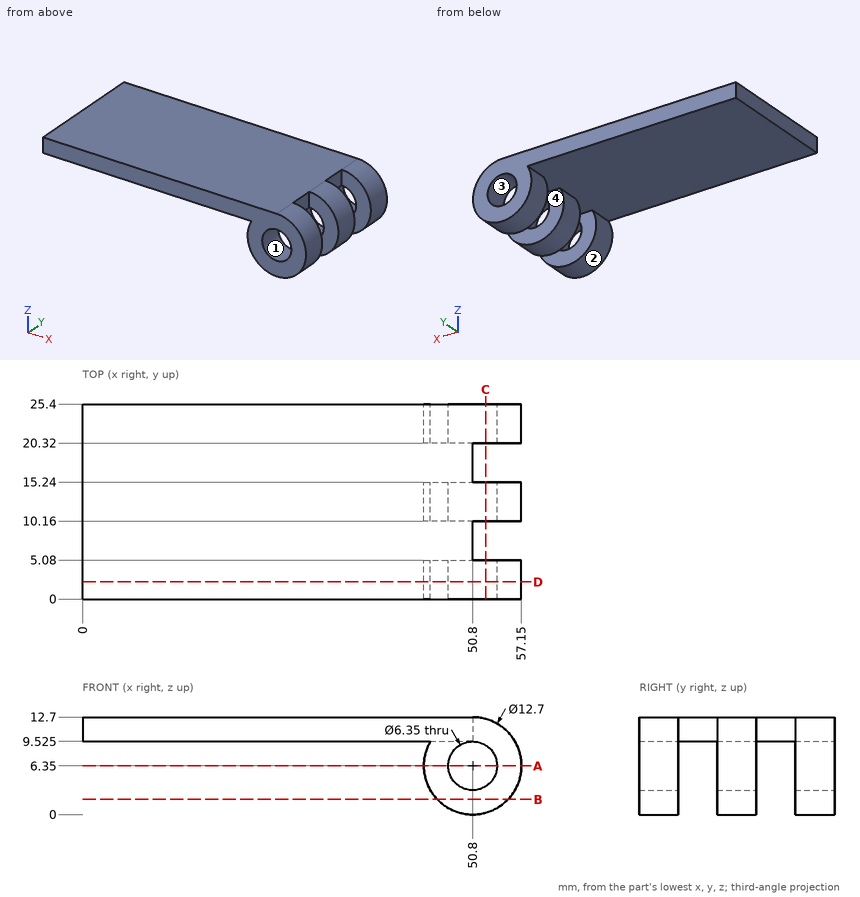
Part print with two shaded views. Sizes in mm from the minimum x, y, z corner. Round coordinates to 2 decimals unless told otherwise and drop trailing zeros. Loops run counter-clockwise (first coordinate to the right, second up) from the corner with the lowest first, then second, coordinate; pieces in that order, holes last.
Item 1: Saw through at D-D (y = 2.25). List the corners of the cut face in (x, z) (3 decimals), then the cut area to 3 significant figures.
Item 2: Saw through at C-C (x = 52.5). List the corners of the cut face in (y, z), then the cut area to 3 significant figures.
Item 3: Drill centre lines: line 1 along X through (y, z) = (3.5, 6.35) (3 decimals); line 2 along Z through (x, y) = (9, 6) (3 decimals); line 3 along X through (y, z) = (24, 9). Where is each one in solid material? Low to high.
Item 4: Saw through at A-A (z = 6.35). List the corners of the cut face in (x, y) (3 decimals).
Item 5: Pin check, flat tips, straight feed: P1, Ø4, axis at x = 45, z = 4.5, coming from the -Y side; P2, Ø1, axis at y = 6.5, z = 11.5, coming from the +X side; P3, Ø4, axis at y = 12, z = 6.5, coming from the -X side; P4, Ø4, axis at y = 15.5, z = 3, coming from the -X side. Stop position of each tip, or through.
Item 6: Two-plate mould, pull along X, no slides. Class the marked faces 1, 2, 3 and 4: released by +X, released by -X, zero draft, split by the parting line, or undercut.
Item 7: Saw through at B-B (z = 2). List the corners of the cut face in (x, y).
Worked answers:
1. outline: (0, 9.525) - (45.301, 9.525) arc R6.35 ccw (long way) to (50.8, 12.7) - (0, 12.7) - close; hole circle Ø6.35 at (50.8, 6.35)
1. area: 244 mm2
2. outline: (0, 0.23) - (5.08, 0.23) - (5.08, 3.67) - (0, 3.67) - close; (0, 9.03) - (5.08, 9.03) - (5.08, 12.47) - (0, 12.47) - close; (10.16, 0.23) - (15.24, 0.23) - (15.24, 3.67) - (10.16, 3.67) - close; (10.16, 9.03) - (15.24, 9.03) - (15.24, 12.47) - (10.16, 12.47) - close; (20.32, 0.23) - (25.4, 0.23) - (25.4, 3.67) - (20.32, 3.67) - close; (20.32, 9.03) - (25.4, 9.03) - (25.4, 12.47) - (20.32, 12.47) - close
2. area: 105 mm2
3. line 1: x = 44.45 to 47.625, 53.975 to 57.15
3. line 2: z = 9.525 to 12.7
3. line 3: x = 45.03 to 49.05, 52.55 to 56.57
4. outline: (44.45, 0) - (47.625, 0) - (47.625, 5.08) - (44.45, 5.08) - close; (44.45, 10.16) - (47.625, 10.16) - (47.625, 15.24) - (44.45, 15.24) - close; (44.45, 20.32) - (47.625, 20.32) - (47.625, 25.4) - (44.45, 25.4) - close; (53.975, 0) - (57.15, 0) - (57.15, 5.08) - (53.975, 5.08) - close; (53.975, 10.16) - (57.15, 10.16) - (57.15, 15.24) - (53.975, 15.24) - close; (53.975, 20.32) - (57.15, 20.32) - (57.15, 25.4) - (53.975, 25.4) - close
5. P1: stops at y = 0
5. P2: stops at x = 50.8
5. P3: stops at x = 44.45
5. P4: stops at x = 44.6
6. face 1: undercut
6. face 2: split by the parting line
6. face 3: undercut
6. face 4: zero draft
7. outline: (46.17, 0) - (55.43, 0) - (55.43, 5.08) - (46.17, 5.08) - close; (46.17, 10.16) - (55.43, 10.16) - (55.43, 15.24) - (46.17, 15.24) - close; (46.17, 20.32) - (55.43, 20.32) - (55.43, 25.4) - (46.17, 25.4) - close
